Build history of the part. All positions in model axes, mm. Face numbers are marked on the shaded views. Give positions to 0.01 mm unless a question says otherwise; leave off trailing zeros. Loops run counter-clockwise (first coordinate to the right, second up) from the corner with the lowest first, then second, coordinate; pieces in that order, holes last. Notation, with made-up numbers: (54.25, 86) -> (79.25, 86) arc R18 cw to (79.25, 93) -> close; hole circle Ø1 at (2.25, 24). An arc over 180 degrees is marked (long way). Answer as a JSON object with one key per item and string values. Group by question number.
Q1. Band-saw the part on A-A, the plane y = 1. Write the cut outline in (x, z).
Q2. Two-plate mould, pull along X, no slides. Class the marked faces 1, 2 and 3: pulls with the +X half, pulls with the -X half, needs draft (parallel to the pull), parting line crosses it, or undercut.
Q3. Band-saw the part on B-B, the plane x = -9. Write the cut outline in (y, z), plus the area to 3 significant figures.
Q4. Wall check: probe 1 along Z at (x, y) = (-14.5, 14); probe 2 along X at (y, z) = (11.5, 10); probe 3 along X at (y, z) = (5.5, 10.25). Give the ranges that are in metal, low to high. Write a range as from..to.
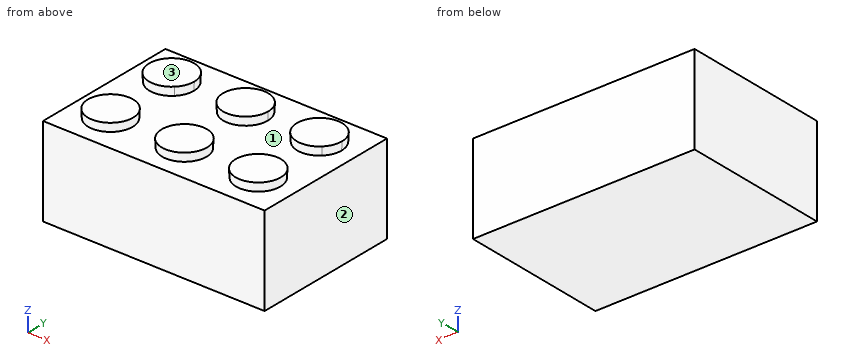
from build123d import *

# Parameters (mm, degrees)
F0_W     = 24
F0_H     = 16
F1_DEPTH = 9.6
F2_R     = 2.4
F3_DEPTH = 0.9
F3_TAPER = -3


with BuildPart() as f1:
    # F0 (on Top) → F1 (new body)
    with BuildSketch(Plane.XY):
        with Locations((-12, 8)):
            Rectangle(F0_W, F0_H)
    extrude(amount=F1_DEPTH)

    # F2 (on face) → F3 (join, symmetric)
    with BuildSketch(Plane.XY.offset(9.6)):
        with Locations((-19.9995, 4)):
            Circle(F2_R)
        with Locations((-11.9985, 4)):
            Circle(F2_R)
        with Locations((-3.999, 4)):
            Circle(F2_R)
        with BuildLine():
            ThreePointArc((-5.695844103, 13.6972684201), (-5.6962684201, 10.303155897), (-2.302155897, 10.3027315799))
            Line((-2.302155897, 10.3027315799), (-5.695844103, 13.6972684201))
        make_face()
        with BuildLine():
            Line((-5.695844103, 13.6972684201), (-2.302155897, 10.3027315799))
            ThreePointArc((-2.302155897, 10.3027315799), (-1.781746536, 11.0814211649), (-1.599, 12))
            ThreePointArc((-1.599, 12), (-3.0804211649, 14.217253464), (-5.695844103, 13.6972684201))
        make_face()
        with BuildLine():
            Line((-21.6966623309, 13.6969502121), (-18.3023376691, 10.3030497879))
            ThreePointArc((-18.3023376691, 10.3030497879), (-17.7821604236, 11.0816290494), (-17.5995, 12))
            ThreePointArc((-17.5995, 12), (-19.0811290494, 14.2173395764), (-21.6966623309, 13.6969502121))
        make_face()
        with BuildLine():
            ThreePointArc((-21.6966623309, 13.6969502121), (-21.6964502121, 10.3028376691), (-18.3023376691, 10.3030497879))
            Line((-18.3023376691, 10.3030497879), (-21.6966623309, 13.6969502121))
        make_face()
        with BuildLine():
            Line((-10.3013376691, 13.6969502121), (-13.6956623309, 10.3030497879))
            ThreePointArc((-13.6956623309, 10.3030497879), (-11.0801290494, 9.7826604236), (-9.5985, 12))
            ThreePointArc((-9.5985, 12), (-9.7811604236, 12.9183709506), (-10.3013376691, 13.6969502121))
        make_face()
        with BuildLine():
            ThreePointArc((-10.3013376691, 13.6969502121), (-13.6954502121, 13.6971623309), (-13.6956623309, 10.3030497879))
            Line((-13.6956623309, 10.3030497879), (-10.3013376691, 13.6969502121))
        make_face()
    extrude(amount=F3_DEPTH, both=True, taper=F3_TAPER)


solid = f1.part
Worked answers:
{
 "1": {"outline": "(-24, 0) -> (0, 0) -> (0, 9.6) -> (-24, 9.6) -> close"},
 "2": {"face 1": "undercut", "face 2": "pulls with the +X half", "face 3": "needs draft"},
 "3": {"outline": "(0, 0) -> (16, 0) -> (16, 9.6) -> (0, 9.6) -> close", "area": "154 mm2"},
 "4": {"probe 1": "0..9.6", "probe 2": "-22.37..-17.63, -14.37..-9.63, -6.37..-1.63", "probe 3": "-21.92..-18.08, -13.92..-10.08, -5.92..-2.08"}
}
